Design review of the part shown in the three views and the two pictorial views. Dimensions are in mm from the part's minimum x, y and z. A direction names the side the tool comes from. Round coordinates to 2 decimals unless told otherwise and drop trailing zeros. Order: outer loops, then holes, each group sorted by start corner. A loop starts at its lowest first (then second) coordinate and runs counter-clockwise, first axis right, second up. Notation, with made-up numbers: (17, -8) - (49, -8) arc R22 cw to (49, 29) - close; hole circle Ø6 at (89.25, 25.5). An arc over 180 degrees is marked (long way). One line per item, written item: value.
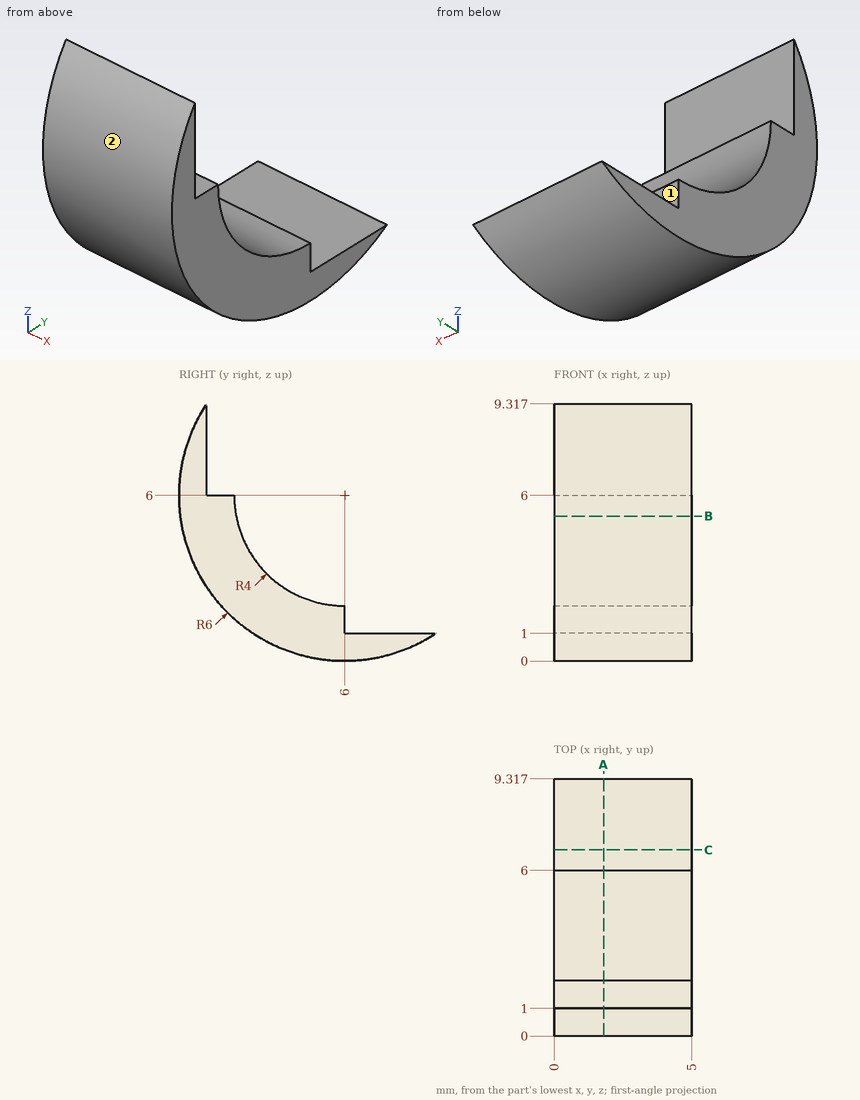
Item 1: Take a section at A-A (x = 1.8). Write out the cut boundary in (y, z).
Returned:
outline: (1, 6) - (1, 9.32) arc R6 ccw to (9.32, 1) - (6, 1) - (6, 2) arc R4 cw to (2, 6) - close
Item 2: For P1, Ø1, axis at x = 3.5, y = 8, coming from the +Z side; P2, Ø2, axis at x = 4, y = 3, coming from the -Z side; P3, Ø1, axis at y = 1.5, z = 1, coming from the +X side, all flat-tipped, find the tip position at first contact; note any pin that passes through.
Returned:
P1: z = 1
P2: z = 0.34
P3: through
Item 3: Wall thickness on line 1 (Y direction, x = 4.75, z = 2.5) (1 decimal); line 2 (Z direction, x = 1.05, y = 7.25); line 3 (Y direction, x = 2.6, z = 5.5): over which ranges is each line inside the solid? List them lowest first.
Returned:
line 1: 1.1 to 4.1
line 2: 0.13 to 1
line 3: 0.02 to 2.03
Item 4: Machinability: for the marked faces 1 and 2, which of the approach directions +Z, -Z, +X, -X, +Y, -Y give a long, thin tool a straight path to every point of the face, cutting with its end or side? Answer none if there is none.
Returned:
face 1: +Z, +X, -X, +Y
face 2: +X, -X
Item 5: Take a section at C-C (y = 6.75). Write out the cut boundary in (x, z).
Returned:
outline: (0, 0.05) - (5, 0.05) - (5, 1) - (0, 1) - close
Item 6: Take a section at B-B (z = 5.25). Write out the cut boundary in (x, y), plus the area to 3 significant figures.
Returned:
outline: (0, 0.05) - (5, 0.05) - (5, 2.07) - (0, 2.07) - close
area: 10.1 mm^2
